```python
from build123d import *

# Parameters (mm, degrees)
SKETCH2_R           = 11.5
BOSS_EXTRUDE1_DEPTH = 116
SKETCH3_R           = 4.45
BOSS_EXTRUDE2_DEPTH = 15
CUT_EXTRUDE1_DEPTH  = 10


with BuildPart() as part:
    # Sketch2 → Boss-Extrude1 (new body)
    with BuildSketch(Plane.XY):
        Circle(SKETCH2_R)
    extrude(amount=-BOSS_EXTRUDE1_DEPTH)

    # Sketch3 → Boss-Extrude2 (add)
    with BuildSketch(Plane(origin=(0, 0, -116), x_dir=(-1, 0, 0), z_dir=(0, 0, -1))):
        Circle(SKETCH3_R)
    extrude(amount=BOSS_EXTRUDE2_DEPTH)

    # Sketch1 → Cut-Extrude1 (cut)
    with BuildSketch(Plane.XY):
        with BuildLine():
            Line((2.051104302, -1.567413373), (-2.047676004, -1.567413373))
            ThreePointArc((-2.047676004, -1.567413373), (-2.598285851, 0.032586627), (-2.047676004, 1.632586627))
            Line((-2.047676004, 1.632586627), (2.051104302, 1.632586627))
            ThreePointArc((2.051104302, 1.632586627), (2.601714149, 0.032586627), (2.051104302, -1.567413373))
        make_face()
    extrude(amount=-CUT_EXTRUDE1_DEPTH, mode=Mode.SUBTRACT)


solid = part.part
```
Geometry check sheet. Reference: the model listing, model coordinates, mm. A direction names the side the tool comes from. Round coordinates to 2 decimals unless told otherwise and drop trailing zeros. Loops run counter-clockwise (first coordinate to the right, second up) from the corner with the lowest first, then second, coordinate; pieces in that order, holes last. Notation, with made-up numbers: M -6,63 L -2,63 A27 ccw -2,100 Z; hole C 46,-13.5 d10. An arc over 180 degrees is marked long. Return JSON: item names as keys, results as strings. Group by question number.
(1) Section check D-D, the plane y = -10. Enter the section's corners in (x, z), and give its area (3 significant figures).
(2) Set-up check for faces 4 (the face through (-2.6, 0, -4.9)), 5 (the face through (-1.5, 11.4, -57.2)): record each of +Z, -Z, +X, -X, +Y, -Y from which the full face is reachable in a straight line by a thin tool's end or side.
(3) Section check B-B, the plane y = 0. Enter the section's corners in (x, z).
(4) Go/stop test with flat-tipped pins: pin 1 (8 mm diameter, centred on x = 4.5, z = -44.5, fed in from +Y); pin 2 (5 mm diameter, centred on x = -8, z = -70.5, fed in from -Y); pin 3 (5 mm diameter, centred on y = 8.5, z = -90, fed in from -X). Record where each tip stops, or that it passes through.
(5) Section check C-C, the plane z = -86.5. Enter the section's corners in (x, y), and give its area (3 significant figures).
(6) Scan lines: line 1 along Z through (x, y) = (-10.5, 2.25); line 2 along X through (y, z) = (0.75, -92.5); line 3 along Y through (x, z) = (9, -113). Record each from-to range of solid material in increasing order. Write a range as [from, to].
(7) Section check A-A, the plane x = 0. Enter the section's corners in (y, z).
(8) Mould release check, pull along X, two halves, no side actions. Record for faces 1 (the face through (0, -1.567, -5)), 2 (the face through (0.965, -4.344, -123.395)), 3 (the face through (5, 0, -116)): pulls with the +X half, pulls with the -X half, needs draft (parallel to the pull), parting line crosses it, or undercut.
Data:
{
 "1": {"outline": "M -5.68,-116 L 5.68,-116 L 5.68,0 L -5.68,0 Z", "area": "1,320 mm²"},
 "2": {"face 4": "+Z", "face 5": "+Z, -Z"},
 "3": {"outline": "M -11.5,-116 L -4.45,-116 L -4.45,-131 L 4.45,-131 L 4.45,-116 L 11.5,-116 L 11.5,0 L 2.6,0 L 2.6,-10 L -2.6,-10 L -2.6,0 L -11.5,0 Z"},
 "4": {"pin 1": "y = 11.49", "pin 2": "y = -10.1", "pin 3": "x = -9.81"},
 "5": {"outline": "C 0,0 d23", "area": "415 mm²"},
 "6": {"line 1": "[-116, 0]", "line 2": "[-11.48, 11.48]", "line 3": "[-7.16, 7.16]"},
 "7": {"outline": "M -11.5,-116 L -4.45,-116 L -4.45,-131 L 4.45,-131 L 4.45,-116 L 11.5,-116 L 11.5,0 L 1.63,0 L 1.63,-10 L -1.57,-10 L -1.57,0 L -11.5,0 Z"},
 "8": {"face 1": "undercut", "face 2": "parting line crosses it", "face 3": "needs draft"}
}
